Design review of the part built by this model. Coordinates are the model's own, in mm. A direction names the side the tool comes from. Coordinates: 2 decimals unless noted, no trailing zeros. Order: outer loops, then holes, each group sorted by start corner. A loop starts at its lowest first (then second) coordinate and runs counter-clockwise, first axis right, second up. Notation, with made-up numbers: M -9.75,15 L -2.75,15 A29 ccw -2.75,48 Z; hole C 58.5,-22.5 d6. An arc over 180 degrees is marked long. Answer as a JSON object with one key per item and string values.
from build123d import *

# Parameters (mm, degrees)
BOSS_EXTRUDE1_DEPTH = 38
SHELL2_T            = -2
CUT_EXTRUDE2_DEPTH  = 1
CUT_EXTRUDE3_START  = -38
CUT_EXTRUDE3_DEPTH  = 1
SKETCH4_W           = 35
SKETCH4_H           = 12.5
CUT_EXTRUDE4_DEPTH  = 1
SKETCH5_W           = 35
SKETCH5_H           = 12.5
CUT_EXTRUDE5_DEPTH  = 1
SKETCH7_W           = 35
SKETCH7_H           = 12.5
CUT_EXTRUDE7_DEPTH  = 1
SKETCH8_W           = 35
SKETCH8_H           = 12.5
CUT_EXTRUDE8_DEPTH  = 1
SKETCH6_R           = 9.8
CUT_EXTRUDE6_DEPTH  = 10
SKETCH9_R           = 2.75
SKETCH9_R_2         = 1.5
BOSS_EXTRUDE2_DEPTH = 6
SKETCH11_W          = 2
SKETCH11_H          = 1.5
BOSS_EXTRUDE5_DEPTH = 18
SKETCH12_W          = 17.8
SKETCH12_H          = 2
CUT_EXTRUDE9_DEPTH  = 18
SKETCH14_R          = 10.8
SKETCH14_R_2        = 9.8
BOSS_EXTRUDE6_DEPTH = 2


with BuildPart() as part:
    # Sketch1 → Boss-Extrude1 (new body)
    with BuildSketch(Plane.XY):
        Polygon((-7.75, -13.423393759), (7.75, -13.423393759), (15.5, 0), (7.75, 13.423393759), (-7.75, 13.423393759), (-15.5, 0), align=None)
        Polygon((23.25, 13.423393759), (15.5, 0), (7.75, 13.423393759), align=None)
        Polygon((38.75, 13.423393759), (23.25, 13.423393759), (15.5, 0), (23.25, -13.423393759), (38.75, -13.423393759), (46.5, 0), align=None)
        Polygon((38.75, 13.423393759), (54.25, 13.423393759), (46.5, 0), align=None)
        Polygon((69.75, 13.423393759), (54.25, 13.423393759), (46.5, 0), (54.25, -13.423393759), (69.75, -13.423393759), (77.5, 0), align=None)
        Polygon((69.75, 13.423393759), (85.25, 13.423393759), (77.5, 0), align=None)
        Polygon((100.75, 13.423393759), (85.25, 13.423393759), (77.5, 0), (85.25, -13.423393759), (100.75, -13.423393759), (108.5, 0), align=None)
    extrude(amount=BOSS_EXTRUDE1_DEPTH)

    # Shell2
    shell2_openings = [part.faces().sort_by_distance(p)[0] for p in [
        (93, -13.423393759, 19),
        (81.375, -6.711696879, 19),
        (73.625, -6.711696879, 19),
        (62, -13.423393759, 19),
        (50.375, -6.711696879, 19),
        (42.625, -6.711696879, 19),
        (31, -13.423393759, 19),
        (19.375, -6.711696879, 19),
        (11.625, -6.711696879, 19),
        (0, -13.423393759, 19),
    ]]
    offset(amount=SHELL2_T, openings=shell2_openings, kind=Kind.INTERSECTION)

    # Sketch3 → Cut-Extrude2 (cut)
    with BuildSketch(Plane.XY.offset(38)):
        Polygon((13.767949192, 0), (6.883974596, 11.923393759), (-6.883974596, 11.923393759), (-13.767949192, 0), (-6.883974596, -11.923393759), (6.883974596, -11.923393759), align=None)
        Polygon((44.767949192, 0), (37.883974596, 11.923393759), (24.116025404, 11.923393759), (17.232050808, 0), (24.116025404, -11.923393759), (37.883974596, -11.923393759), align=None)
        Polygon((75.767949192, 0), (68.883974596, 11.923393759), (55.116025404, 11.923393759), (48.232050808, 0), (55.116025404, -11.923393759), (68.883974596, -11.923393759), align=None)
        Polygon((106.767949192, 0), (99.883974596, 11.923393759), (86.116025404, 11.923393759), (79.232050808, 0), (86.116025404, -11.923393759), (99.883974596, -11.923393759), align=None)
    extrude(amount=-CUT_EXTRUDE2_DEPTH, mode=Mode.SUBTRACT)

    # Sketch3<2> → Cut-Extrude3 (cut)
    with BuildSketch(Plane.XY.offset(38).offset(CUT_EXTRUDE3_START)):
        Polygon((13.767949192, 0), (6.883974596, 11.923393759), (-6.883974596, 11.923393759), (-13.767949192, 0), (-6.883974596, -11.923393759), (6.883974596, -11.923393759), align=None)
        Polygon((44.767949192, 0), (37.883974596, 11.923393759), (24.116025404, 11.923393759), (17.232050808, 0), (24.116025404, -11.923393759), (37.883974596, -11.923393759), align=None)
        Polygon((75.767949192, 0), (68.883974596, 11.923393759), (55.116025404, 11.923393759), (48.232050808, 0), (55.116025404, -11.923393759), (68.883974596, -11.923393759), align=None)
        Polygon((106.767949192, 0), (99.883974596, 11.923393759), (86.116025404, 11.923393759), (79.232050808, 0), (86.116025404, -11.923393759), (99.883974596, -11.923393759), align=None)
    extrude(amount=CUT_EXTRUDE3_DEPTH, mode=Mode.SUBTRACT)

    # Sketch4 → Cut-Extrude4 (cut)
    with BuildSketch(Plane(origin=(81.375, 46.981878155, 0), x_dir=(0, 0, -1), z_dir=(0.866025404, 0.5, 0))):
        with Locations((-19, -46.5)):
            Rectangle(SKETCH4_W, SKETCH4_H)
    extrude(amount=-CUT_EXTRUDE4_DEPTH, mode=Mode.SUBTRACT)

    # Sketch5 → Cut-Extrude5 (cut)
    with BuildSketch(Plane(origin=(-11.625, 6.711696879, 0), x_dir=(0, 0, 1), z_dir=(-0.866025404, 0.5, 0))):
        with Locations((19, 0)):
            Rectangle(SKETCH5_W, SKETCH5_H)
    extrude(amount=-CUT_EXTRUDE5_DEPTH, mode=Mode.SUBTRACT)

    # Sketch7 → Cut-Extrude7 (cut)
    with BuildSketch(Plane(origin=(-11.625, -6.711696879, 0), x_dir=(0, 0, 1), z_dir=(-0.866025404, -0.5, 0))):
        with Locations((19, 0)):
            Rectangle(SKETCH7_W, SKETCH7_H)
    extrude(amount=-CUT_EXTRUDE7_DEPTH, mode=Mode.SUBTRACT)

    # Sketch8 → Cut-Extrude8 (cut)
    with BuildSketch(Plane(origin=(81.375, -46.981878155, 0), x_dir=(0, 0, -1), z_dir=(0.866025404, -0.5, 0))):
        with Locations((-19, 46.5)):
            Rectangle(SKETCH8_W, SKETCH8_H)
    extrude(amount=-CUT_EXTRUDE8_DEPTH, mode=Mode.SUBTRACT)

    # Sketch6 → Cut-Extrude6 (cut)
    with BuildSketch(Plane(origin=(0, 13.423393759, 0), x_dir=(1, 0, 0), z_dir=(0, 1, 0))):
        with Locations((6.5, -19)):
            Circle(SKETCH6_R)
        with Locations((29.5, -19)):
            Circle(SKETCH6_R)
        with Locations((63.5, -19)):
            Circle(SKETCH6_R)
        with Locations((86.5, -19)):
            Circle(SKETCH6_R)
    extrude(amount=-CUT_EXTRUDE6_DEPTH, mode=Mode.SUBTRACT)

    # Sketch9 → Boss-Extrude2 (add)
    with BuildSketch(Plane.XZ.offset(-11.423393759)):
        with Locations((-0.5, 31)):
            Circle(SKETCH9_R)
        with Locations((-0.5, 31)):
            Circle(SKETCH9_R_2, mode=Mode.SUBTRACT)
        with Locations((-0.5, 7)):
            Circle(SKETCH9_R)
        with Locations((-0.5, 7)):
            Circle(SKETCH9_R_2, mode=Mode.SUBTRACT)
        with Locations((93.5, 31)):
            Circle(SKETCH9_R)
        with Locations((93.5, 31)):
            Circle(SKETCH9_R_2, mode=Mode.SUBTRACT)
        with Locations((93.5, 7)):
            Circle(SKETCH9_R)
        with Locations((93.5, 7)):
            Circle(SKETCH9_R_2, mode=Mode.SUBTRACT)
    extrude(amount=BOSS_EXTRUDE2_DEPTH)

    # Sketch11 → Boss-Extrude5 (add)
    with BuildSketch(Plane.XZ.offset(-11.423393759)):
        with Locations((52.1, 35.25)):
            Rectangle(SKETCH11_W, SKETCH11_H)
        with Locations((71.9, 35.25)):
            Rectangle(SKETCH11_W, SKETCH11_H)
    extrude(amount=BOSS_EXTRUDE5_DEPTH)

    # Sketch12 → Cut-Extrude9 (cut)
    with BuildSketch(Plane.XZ.offset(-11.423393759)):
        with Locations((62, 35.5)):
            Rectangle(SKETCH12_W, SKETCH12_H)
    extrude(amount=CUT_EXTRUDE9_DEPTH, mode=Mode.SUBTRACT)

    # Sketch14 → Boss-Extrude6 (add)
    with BuildSketch(Plane.XZ.offset(-11.423393759)):
        with Locations((6.5, 19)):
            Circle(SKETCH14_R)
        with Locations((6.5, 19)):
            Circle(SKETCH14_R_2, mode=Mode.SUBTRACT)
        with Locations((29.5, 19)):
            Circle(SKETCH14_R)
        with Locations((29.5, 19)):
            Circle(SKETCH14_R_2, mode=Mode.SUBTRACT)
        with Locations((63.5, 19)):
            Circle(SKETCH14_R)
        with Locations((63.5, 19)):
            Circle(SKETCH14_R_2, mode=Mode.SUBTRACT)
        with Locations((86.5, 19)):
            Circle(SKETCH14_R)
        with Locations((86.5, 19)):
            Circle(SKETCH14_R_2, mode=Mode.SUBTRACT)
    extrude(amount=BOSS_EXTRUDE6_DEPTH)


solid = part.part
1) Tool access review of faces 4 (the flat face through (102.26, -6.81, 18.76)), 5 (the flat face through (42.57, -6.81, 36.99)), 6 (the cylindrical face through (-0.858, 8.465, 33.727)), 7 (the cylindrical face through (38.553, 11.451, 15.247)), 8 (the flat face through (41.278, -6.045, 37.507)): name each direction out of +Z, -Z, +X, -X, +Y, -Y from which nothing blocks a thin tool from reaching the whole face with its end or side.
Taken from the geometry:
{"face 4": "none", "face 5": "+Z, -Z, -Y", "face 6": "-Y", "face 7": "+Y, -Y", "face 8": "+Z"}
2) Add section A-A (x = 29.5). State the section outline as (y, z) points, and give its area (3 significant figures).
Taken from the geometry:
{"outline": "M -13.42,0 L -11.92,0 L -11.92,1 L 11.92,1 L 11.92,0 L 13.42,0 L 13.42,9.2 L 9.42,9.2 L 9.42,8.2 L 11.42,8.2 L 11.42,2 L -13.42,2 Z; M -13.42,36 L 11.42,36 L 11.42,29.8 L 9.42,29.8 L 9.42,28.8 L 13.42,28.8 L 13.42,38 L 11.92,38 L 11.92,37 L -11.92,37 L -11.92,38 L -13.42,38 Z", "area": "92.5 mm2"}
3) Add section B-B (z = 19). Count the separate pieces of the cut face and the enclosed holes in it, and give its area (3 significant figures).
Taken from the geometry:
{"separate pieces": "5", "enclosed holes": "0", "area": "143 mm2"}
4) Insertion check: pin 1 Ø4 at (x, y) = (55, -9.5) entering from +Z; pin 2 Ø3.5 at (x, z) = (93.5, 7.5) entering from -Y; pin 3 Ø1 at (x, z) = (52.5, 9.5) entering from -Y; pin 4 Ø12 at (x, y) = (33.5, 4.5) entering from +Z. Each pin has a flat end and moves straight along its axis. Give the tip position at first contact, or say it passes through.
Taken from the geometry:
{"pin 1": "stops at z = 38", "pin 2": "stops at y = 5.42", "pin 3": "stops at y = 11.42", "pin 4": "stops at z = 37"}
5) To check wall thickness, follow L1, parallel to Z at x = 6.5, y = 11.2; L2, parallel to Z at x = 93.5, y = 7.6; L3, parallel to Z at x = 2, y = -11.5. State the ranges of each line that lie inside material, in increasing order.
Taken from the geometry:
{"L1": "z = 1 to 2, 8.2 to 9.2, 28.8 to 29.8, 36 to 37", "L2": "z = 1 to 2, 4.25 to 5.5, 8.5 to 9.75, 28.25 to 29.5, 32.5 to 33.75, 36 to 37", "L3": "z = 1 to 2, 36 to 37"}
6) Mouldability with a two-part tool opening along X and no side actions: class faces 1 (the flat face through (101.16, -12.71, 17.5)), 2 (the flat face through (103.278, -6.045, 0.493)), 3 (the flat face through (31, -13.423, 1)) as released by +X, released by -X, zero draft, split by the parting line, or undercut.
Taken from the geometry:
{"face 1": "released by +X", "face 2": "undercut", "face 3": "zero draft"}
7) Add section C-C (x = 63.5). State the section outline as (y, z) points.
Taken from the geometry:
{"outline": "M -13.42,0 L -11.92,0 L -11.92,1 L 11.92,1 L 11.92,0 L 13.42,0 L 13.42,9.2 L 9.42,9.2 L 9.42,8.2 L 11.42,8.2 L 11.42,2 L -13.42,2 Z; M -13.42,36 L -6.58,36 L -6.58,36.5 L 11.42,36.5 L 11.42,29.8 L 9.42,29.8 L 9.42,28.8 L 13.42,28.8 L 13.42,38 L 11.92,38 L 11.92,37 L -11.92,37 L -11.92,38 L -13.42,38 Z"}
8) Add section D-D (x = 9). State the section outline as (y, z) points, and give its area (3 significant figures).
Taken from the geometry:
{"outline": "M -11.26,0 L -8.26,0 L -8.26,1 L 8.26,1 L 8.26,0 L 13.42,0 L 13.42,9.52 L 9.42,9.52 L 9.42,8.49 L 11.42,8.49 L 11.42,2 L -11.26,2 Z; M -11.26,36 L 11.42,36 L 11.42,29.51 L 9.42,29.51 L 9.42,28.48 L 13.42,28.48 L 13.42,38 L 8.26,38 L 8.26,37 L -8.26,37 L -8.26,38 L -11.26,38 Z", "area": "99.9 mm2"}
